Part print with two shaded views. Sizes in mm from the minimum x, y, z corner. A direction names the side the tool comes from. Give positions to 0.01 mm unless a question says otherwise; leave off trailing zeros. Loops run counter-clockwise (first coordinate to the right, second up) from the corner with the lowest first, then second, coordinate; pieces in that order, holes last. Notation, with made-up numbers: M 68,78 L 75,78 A34 cw 75,111 Z; hole C 36.5,3 d5. An arc over 180 degrees is marked long. Answer as a JSON object with one key per item and string values. Group by question number.
1. Slice it at D-D (x = 65). List the corners of the cut face in (y, z).
2. Slice it at B-B (x = 42). List the corners of the cut face in (y, z) (1 decimal), then the cut area to 3 significant figures.
3. Slice it at A-A (z = 47). List the corners of the cut face in (x, y).
4. Mould opens along X. For the marked faces 1, 2 and 3 say: released by +X, released by -X, zero draft, split by the parting line, or undercut.
5. Drill centre lines: line 1 along Z through (x, y) = (57, 36.5); line 2 along Y through (x, z) = (78.5, 30); line 3 along X through (y, z) = (41.5, 45). Where is each one in solid material? Low to high. Write a range as [from, to].
6. Drop a flat-ended pin along its axis: pin 1 Ø6 at (x, y) = (73.5, 13) entering from +Z. Give the stop position or say it passes through.
7. 3-axis set-ups, long thin cutter, end or side, ignore diameter. For the marked faces 4 and 5: which of +Z, -Z, +X, -X, +Y, -Y reach the whole face in a straight line?
8. Slice it at C-C (y = 21). List the corners of the cut face in (x, z) (1 decimal), then the cut area to 3 significant figures.
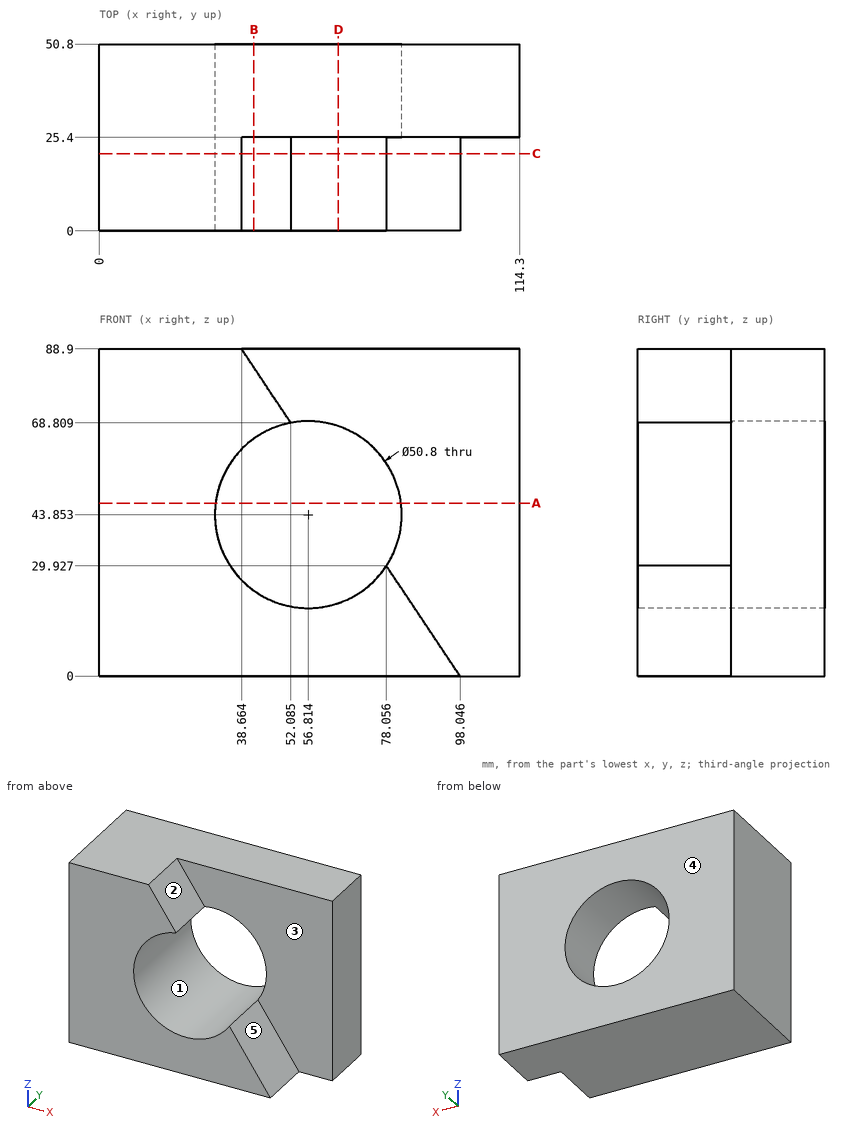
Established:
{
 "1": {"outline": "M 0,0 L 50.8,0 L 50.8,19.81 L 0,19.81 Z; M 25.4,67.9 L 50.8,67.9 L 50.8,88.9 L 25.4,88.9 Z"},
 "2": {"outline": "M 0,0 L 50.8,0 L 50.8,23.2 L 0,23.2 Z; M 0,64.5 L 50.8,64.5 L 50.8,88.9 L 25.4,88.9 L 25.4,83.9 L 0,83.9 Z", "area": "2,290 mm^2"},
 "3": {"outline": "M 0,0 L 31.61,0 L 31.61,50.8 L 0,50.8 Z; M 82.02,25.4 L 114.3,25.4 L 114.3,50.8 L 82.02,50.8 Z"},
 "4": {"face 1": "undercut", "face 2": "released by +X", "face 3": "zero draft"},
 "5": {"line 1": "z = [0, 18.45], [69.25, 88.9]", "line 2": "y = [25.4, 50.8]", "line 3": "x = [0, 31.44], [82.19, 114.3]"},
 "6": {"pin 1": "stops at z = 27.8"},
 "7": {"face 4": "+Z, -Z, +X, -X, +Y", "face 5": "+Z, +X, -Y"},
 "8": {"outline": "M 0,0 L 98,0 L 78.1,29.9 A25.4 cw long 52.1,68.8 L 38.7,88.9 L 0,88.9 Z", "area": "4,570 mm^2"}
}
